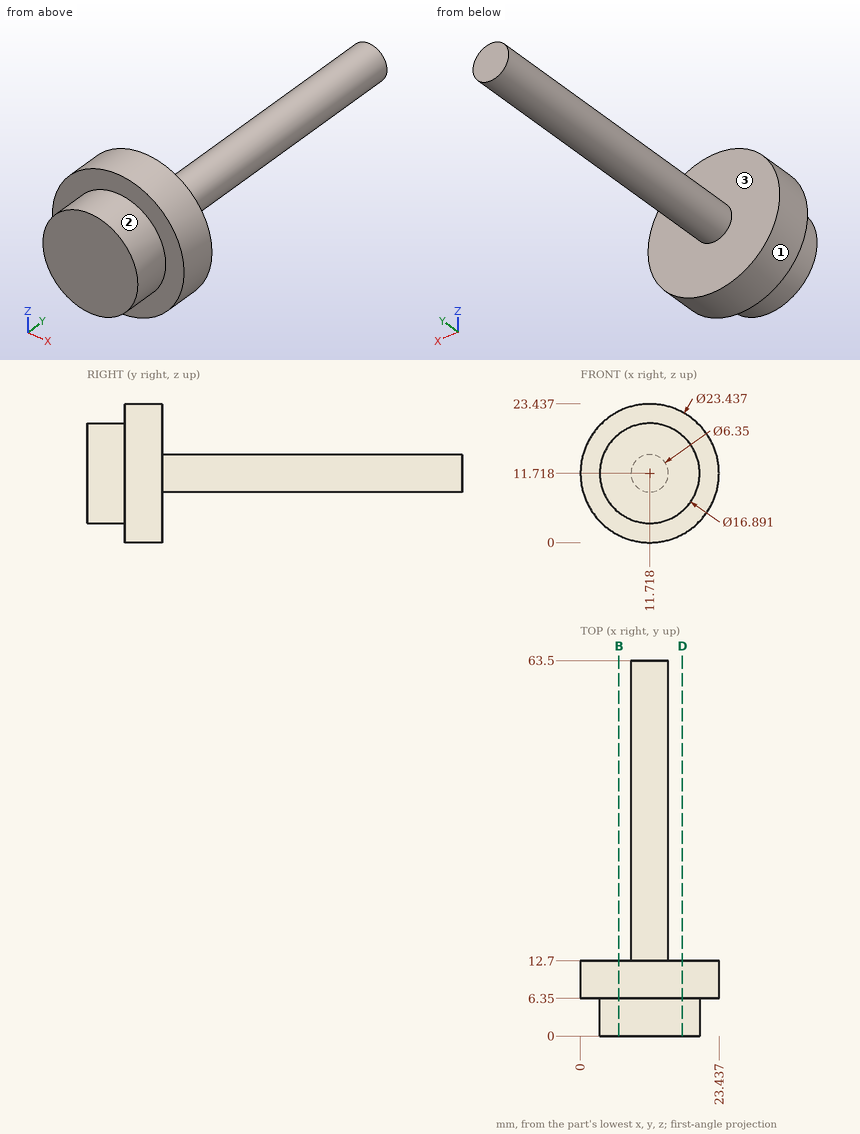
For this review, use the dimensioned drawing (mm, ordinates from the lowest corner) and the shaded views. A direction names the side the tool comes from. Coordinates: 2 decimals unless noted, no trailing zeros. Loops run counter-clockwise (first coordinate to the right, second up) from the corner with the lowest first, then second, coordinate; pieces in that order, holes last. Notation, with made-up numbers: M -27.5,67 L -21.5,67 A33 cw -21.5,97 Z; hole C 9,-39 d1. An arc over 180 degrees is marked long. Answer as CSV lines item,"result".
Item 1: Add section B-B on x = 6.5. State the section outline as (y, z) points.
Answer list:
outline,"M 0,5.08 L 6.35,5.08 L 6.35,1.23 L 12.7,1.23 L 12.7,22.21 L 6.35,22.21 L 6.35,18.36 L 0,18.36 Z"
Item 2: For probe 1 along Y at (x, z) = (10.75, 19.5); probe 2 along Y at (x, z) = (17, 21); probe 3 along X at (y, z) = (52, 12.5) (1 decimal), list the stretches that pass through material, from the lowest coordinate up.
Answer list:
probe 1,"0 to 12.7"
probe 2,"6.35 to 12.7"
probe 3,"8.6 to 14.8"
Item 3: For P1, Ø1.5, axis at x = 4, z = 20, coming from the +Y side; P2, Ø5, axis at y = 13, z = 4.5, coming from the -X side; P3, Ø12, axis at x = 6, z = 4, coming from the -Y side; P4, Ø2, axis at x = 3, y = 10.5, coming from the -Z side, all flat-tipped, find the tip position at first contact; note any pin that passes through.
Answer list:
P1,"y = 12.7"
P2,"x = 1"
P3,"y = 0"
P4,"z = 2.9"
Item 4: Machinability: for the marked faces 1, 2 and 3, which of the approach directions +Z, -Z, +X, -X, +Y, -Y give a long, thin tool a straight path to every point of the face, cutting with its end or side? Answer none if there is none.
Answer list:
face 1,"+Y, -Y"
face 2,"-Y"
face 3,"+Y"
Item 5: Add section D-D on x = 17.25. State the section outline as (y, z) points, plus the area to 3 significant figures.
Answer list:
outline,"M 0,5.34 L 6.35,5.34 L 6.35,1.39 L 12.7,1.39 L 12.7,22.05 L 6.35,22.05 L 6.35,18.1 L 0,18.1 Z"
area,"212 mm²"
